Input: part model. Units: mm. Frame: model coordinates. Give positions to 0.01 mm unless a question says otherwise; leave off trailing zeros. Write each loop counter-clockwise with the first axis right and the second up, starting at its lowest first coordinate (ties: lowest second). Pieces come first, ordered by that corner, then holes. Notation, with made-up numbers: (-16.5, 9) - (5.5, 9) arc R29 cw to (5.5, 42) - close; hole circle Ø4 at (-0.75, 10). An arc over 180 degrees is marked (long way). Use a Markdown table: item, result. Add a question column.
1. Section query D-D, the plane z = 0.7. Count the separate pieces of the cut face and the enclosed holes in it, plus the area to 3 significant figures.
2. Pin query (flat end, axial travel): pin 1 (1.5 mm diameter, centred on y = 139.5, z = 2, fed in from +X); pin 2 (0.9 mm diameter, centred on y = 87, z = 1, fed in from -X); pin 3 (0.9 mm diameter, centred on x = -87.5, z = 1, fed in from -Y). Return the tip coordinate at first contact, or that it passes through.
3. Section query B-B, the plane y = -133. Return loops of the section in (x, z), plus the area to 3 significant figures.
4. Material intervals for probe 1 along X at (y, z) = (-67, 2.1); probe 2 along Y at (x, z) = (-65, 1.2); probe 3 along Y at (x, z) = (20, 1.15), sorted ascending.
5. Section query C-C, the plane x = 82.5. Return loops of the section in (y, z).
6. Section query A-A, the plane x = -83. Return loops of the section in (y, z), plus the area to 3 significant figures.
```python
from build123d import *

# Parameters (mm, degrees)
SKETCH_1_R           = 175
EXTRUDE_1_DEPTH      = 3
CUT_EXTRUDE_1_DEPTH  = 3
FILLET_1_R           = 5
FILLET_2_R           = 5
FILLET_3_R           = 5
SKETCH_5_R           = 1.5
CUT_EXTRUDE_4_DEPTH  = 3
SKETCH_6_R           = 1.5
CUT_EXTRUDE_5_DEPTH  = 3
SKETCH_7_W           = 30
SKETCH_7_H           = 108
CUT_EXTRUDE_6_DEPTH  = 3
SKETCH_8_R           = 1.5
CUT_EXTRUDE_7_DEPTH  = 3
SKETCH_9_R           = 1.5
CUT_EXTRUDE_8_DEPTH  = 10
SKETCH_10_R          = 1.6
CUT_EXTRUDE_9_DEPTH  = 10
SKETCH_11_W          = 15
SKETCH_11_H          = 30
CUT_EXTRUDE_10_DEPTH = 10


with BuildPart() as part:
    # ｽｹｯﾁ1 → ﾎﾞｽ - 押し出し1 (new body)
    with BuildSketch(Plane.XY):
        Circle(SKETCH_1_R)
    extrude(amount=EXTRUDE_1_DEPTH)

    # ｽｹｯﾁ2 → ｶｯﾄ - 押し出し1 (cut)
    with BuildSketch(Plane.XY.offset(3)):
        with BuildLine():
            Line((-60, 115), (0, 115))
            Line((0, 115), (0, 175))
            ThreePointArc((0, 175), (-30.465194158, 172.327803749), (-60, 164.392822228))
            Line((-60, 164.392822228), (-60, 115))
        make_face()
        with BuildLine():
            Line((0, 175), (0, 115))
            Line((0, 115), (60, 115))
            Line((60, 115), (60, 164.392822228))
            ThreePointArc((60, 164.392822228), (30.465194158, 172.327803749), (0, 175))
        make_face()
        with BuildLine():
            Line((0, -175), (0, -115))
            Line((0, -115), (-60, -115))
            Line((-60, -115), (-60, -164.392822228))
            ThreePointArc((-60, -164.392822228), (-30.465194158, -172.327803749), (0, -175))
        make_face()
        with BuildLine():
            Line((60, -115), (0, -115))
            Line((0, -115), (0, -175))
            ThreePointArc((0, -175), (30.465194158, -172.327803749), (60, -164.392822228))
            Line((60, -164.392822228), (60, -115))
        make_face()
    extrude(amount=-CUT_EXTRUDE_1_DEPTH, mode=Mode.SUBTRACT)

    # ﾌｨﾚｯﾄ1
    fillet_1_edges = [part.edges().sort_by_distance(p)[0] for p in [
        (-60, 164.392822228, 1.5),
    ]]
    fillet(fillet_1_edges, radius=FILLET_1_R)

    # ﾌｨﾚｯﾄ2
    fillet_2_edges = [part.edges().sort_by_distance(p)[0] for p in [
        (-60, 115, 1.5),
        (60, 164.392822228, 1.5),
        (60, 115, 1.5),
    ]]
    fillet(fillet_2_edges, radius=FILLET_2_R)

    # ﾌｨﾚｯﾄ3
    fillet_3_edges = [part.edges().sort_by_distance(p)[0] for p in [
        (-60, -115, 1.5),
        (60, -115, 1.5),
        (60, -164.392822228, 1.5),
        (-60, -164.392822228, 1.5),
    ]]
    fillet(fillet_3_edges, radius=FILLET_3_R)

    # ｽｹｯﾁ5 → ｶｯﾄ - 押し出し4 (cut)
    with BuildSketch(Plane.XY.offset(3)):
        with Locations((-100, -115)):
            Circle(SKETCH_5_R)
        with Locations((100, -115)):
            Circle(SKETCH_5_R)
        with Locations((100, 115)):
            Circle(SKETCH_5_R)
        with Locations((-100, 115)):
            Circle(SKETCH_5_R)
    extrude(amount=-CUT_EXTRUDE_4_DEPTH, mode=Mode.SUBTRACT)

    # ｽｹｯﾁ6 → ｶｯﾄ - 押し出し5 (cut)
    with BuildSketch(Plane.XY.offset(3)):
        with Locations((-60, 54)):
            Circle(SKETCH_6_R)
        with Locations((60, 54)):
            Circle(SKETCH_6_R)
        with Locations((-60, -54)):
            Circle(SKETCH_6_R)
        with Locations((60, -54)):
            Circle(SKETCH_6_R)
    extrude(amount=-CUT_EXTRUDE_5_DEPTH, mode=Mode.SUBTRACT)

    # ｽｹｯﾁ7 → ｶｯﾄ - 押し出し6 (cut)
    with BuildSketch(Plane.XY.offset(3)):
        with Locations((-85, 0)):
            Rectangle(SKETCH_7_W, SKETCH_7_H)
    extrude(amount=-CUT_EXTRUDE_6_DEPTH, mode=Mode.SUBTRACT)

    # ｽｹｯﾁ8 → ｶｯﾄ - 押し出し7 (cut)
    with BuildSketch(Plane.XY.offset(3)):
        with Locations((-115, -67)):
            Circle(SKETCH_8_R)
        with Locations((-116.822468618, 0)):
            Circle(SKETCH_8_R)
        with Locations((-115, 67)):
            Circle(SKETCH_8_R)
    extrude(amount=-CUT_EXTRUDE_7_DEPTH, mode=Mode.SUBTRACT)

    # ｽｹｯﾁ9 → ｶｯﾄ - 押し出し8 (cut)
    with BuildSketch(Plane.XY.offset(3)):
        with Locations((-65, 37)):
            Circle(SKETCH_9_R)
        with Locations((20, 41)):
            Circle(SKETCH_9_R)
        with Locations((-65, -38)):
            Circle(SKETCH_9_R)
        with Locations((20, -40)):
            Circle(SKETCH_9_R)
    extrude(amount=-CUT_EXTRUDE_8_DEPTH, mode=Mode.SUBTRACT)

    # ｽｹｯﾁ10 → ｶｯﾄ - 押し出し9 (cut)
    with BuildSketch(Plane.XY.offset(3)):
        with Locations((111.643659725, -125.921059639)):
            Circle(SKETCH_10_R)
        with Locations((122.679794489, -115.037952538)):
            Circle(SKETCH_10_R)
        with Locations((168, 7.75)):
            Circle(SKETCH_10_R)
        with Locations((168, -7.75)):
            Circle(SKETCH_10_R)
        with Locations((111.56768007, 125.844011632)):
            Circle(SKETCH_10_R)
        with Locations((122.679794489, 115.037952538)):
            Circle(SKETCH_10_R)
    extrude(amount=-CUT_EXTRUDE_9_DEPTH, mode=Mode.SUBTRACT)

    # ｽｹｯﾁ11 → ｶｯﾄ - 押し出し10 (cut)
    with BuildSketch(Plane.XY.offset(3)):
        with Locations((81.317279836, 81.317279836)):
            Rectangle(SKETCH_11_W, SKETCH_11_H)
        with Locations((81.317279836, -81.317279836)):
            Rectangle(SKETCH_11_W, SKETCH_11_H)
    extrude(amount=-CUT_EXTRUDE_10_DEPTH, mode=Mode.SUBTRACT)


solid = part.part
```
Result sheet:
| question | item | result |
|---|---|---|
| 1 | separate pieces | 1 |
| 1 | enclosed holes | 24 |
| 1 | area | 78,300 mm² |
| 2 | pin 1 | stops at x = 106.65 |
| 2 | pin 2 | stops at x = -152.1 |
| 2 | pin 3 | stops at y = -151.81 |
| 3 | outline | (-113.74, 0) - (-60, 0) - (-60, 3) - (-113.74, 3) - close; (60, 0) - (113.74, 0) - (113.74, 3) - (60, 3) - close |
| 3 | area | 322 mm² |
| 4 | probe 1 | x = -161.67 to -116.5, -113.5 to 73.82, 88.82 to 161.67 |
| 4 | probe 2 | y = -162.08 to -39.5, -36.5 to 35.5, 38.5 to 162.08 |
| 4 | probe 3 | y = -115 to -41.5, -38.5 to 39.5, 42.5 to 115 |
| 5 | outline | (-154.33, 0) - (-96.32, 0) - (-96.32, 3) - (-154.33, 3) - close; (-66.32, 0) - (66.32, 0) - (66.32, 3) - (-66.32, 3) - close; (96.32, 0) - (154.33, 0) - (154.33, 3) - (96.32, 3) - close |
| 6 | outline | (-154.06, 0) - (-54, 0) - (-54, 3) - (-154.06, 3) - close; (54, 0) - (154.06, 0) - (154.06, 3) - (54, 3) - close |
| 6 | area | 600 mm² |
